For this review, take the finished solid that the model builds, in its own axes (mm). Face numbers are marked on the shaded views. A direction names the side the tool comes from. Coordinates: 2 decimals unless noted, no trailing zeros. Order: outer loops, then holes, each group sorted by start corner. A loop starts at its lowest first (then second) coordinate and runs counter-clockwise, first axis right, second up. Notation, with made-up numbers: (3, 64.5) -> (43, 64.5) arc R19 cw to (43, 98.5) -> close; hole circle Ø8 at (87, 21). An arc over 180 degrees is marked (long way). Answer as a JSON object with one key per item and string values. Group by question number.
1) For pin 1 (3 mm diameter, centred on y = 22.5, z = 13.5, fed in from +X); pin 2 (16.5 mm diameter, centred on y = 17, z = -3, fed in from +X); pin 3 (6 mm diameter, centred on x = -4, z = 11, fed in from -Y); pin 4 (10 mm diameter, centred on x = -21, y = 1, fed in from -Z), all flat-tipped, find the tip position at first contact; note any pin that passes through.
2) Draft analysis for pull direction X (two halves, no side actions). For the marked faces 1, 2, 3 and 4, state which applies: +X half, -X half, draft (parallel to the pull), parting line (faces both ways), or undercut.
3) Add section C-C, the plane x = 27. Write out the cut boundary in (y, z), then the cut area to 3 significant figures.
4) Add section D-D, the plane x = 12. Write out the cut boundary in (y, z), then the cut area to 3 significant figures.
5) Add section B-B, the plane y = 15. Write out the cut boundary in (x, z), then the cut area to 3 significant figures.
6) Wall thickness on L1, parallel to X at y = -7, z = 1; L2, parallel to Y at x = 28.25, z = 0; L3, parallel to Y at x = -1, z = 0: over which ranges is each line inside the solid? List them lowest first.
7) Machinability: for the marked faces 5, 6 and 7, which of the approach directions +Z, -Z, +X, -X, +Y, -Y give a long, thin tool a straight path to every point of the face, cutting with its end or side? Answer none if there is none.
8) Add section A-A, the plane z = 0. Write out the cut boundary in (x, y), then the cut area to 3 significant figures.
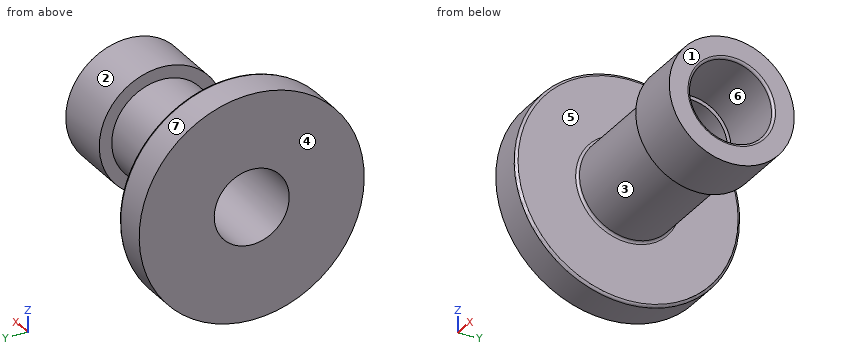
from build123d import *

# Parameters (mm, degrees)
HOLE1_D     = 30
HOLE2_D     = 33
HOLE2_DEPTH = 30
FILLET1_R   = 1


with BuildPart() as part:
    # Sketch1 → Revolve1 (revolve)
    with BuildSketch(Plane.XY, mode=Mode.PRIVATE) as revolve1_sk:
        Polygon((-44.2, 15), (-44.2, 60), (-30, 60), (-30, 35), (20.2, 35), (20.2, 40), (44.2, 40), (44.2, 15), align=None)
    revolve(revolve1_sk.sketch.rotate(Axis((44.2, 15, 0), (-1, 0, 0)), 90), axis=Axis((44.2, 15, 0), (-1, 0, 0)))

    # Hole1 (through all)
    with Locations(Plane(origin=(44.2, 0, 0), x_dir=(0, 0, -1), z_dir=(1, 0, 0))):
        with Locations((0, 15)):
            Hole(HOLE1_D / 2)

    # Hole2
    with Locations(Plane(origin=(44.2, 0, 0), x_dir=(0, 0, -1), z_dir=(1, 0, 0))):
        with Locations((0, 15)):
            Hole(HOLE2_D / 2, depth=HOLE2_DEPTH)

    # Fillet1
    fillet1_edges = [part.edges().sort_by_distance(p)[0] for p in [
        (44.2, 15, -16.5),
        (-30, 15, 20),
        (-30, 15, 45),
    ]]
    fillet(fillet1_edges, radius=FILLET1_R)


solid = part.part
Output values:
{
 "1": {"pin 1": "stops at x = 44.03", "pin 2": "passes through", "pin 3": "stops at y = -3.33", "pin 4": "stops at z = -17.86"},
 "2": {"face 1": "+X half", "face 2": "draft", "face 3": "undercut", "face 4": "-X half"},
 "3": {"outline": "circle Ø50 at (15, 0); hole circle Ø33 at (15, 0)", "area": "1,110 mm²"},
 "4": {"outline": "circle Ø40 at (15, 0); hole circle Ø30 at (15, 0)", "area": "550 mm²"},
 "5": {"outline": "(-44.2, -45) -> (-31, -45) arc R1 ccw to (-30, -44) -> (-30, -21) arc R1 cw to (-29, -20) -> (20.2, -20) -> (20.2, -25) -> (44.2, -25) -> (44.2, -17.5) arc R1 ccw to (43.2, -16.5) -> (14.2, -16.5) -> (14.2, -15) -> (-44.2, -15) -> close; (-44.2, 15) -> (14.2, 15) -> (14.2, 16.5) -> (43.2, 16.5) arc R1 ccw to (44.2, 17.5) -> (44.2, 25) -> (20.2, 25) -> (20.2, 20) -> (-29, 20) arc R1 cw to (-30, 21) -> (-30, 44) arc R1 ccw to (-31, 45) -> (-44.2, 45) -> close", "area": "1,740 mm²"},
 "6": {"L1": "x = -44.2 to -30, 20.2 to 44.2", "L2": "y = -10 to -1.5, 31.5 to 40", "L3": "y = -5 to 0, 30 to 35"},
 "7": {"face 5": "none", "face 6": "+X", "face 7": "+X, -X"},
 "8": {"outline": "(-44.2, -30) -> (-31, -30) arc R1 ccw to (-30, -29) -> (-30, -6) arc R1 cw to (-29, -5) -> (20.2, -5) -> (20.2, -10) -> (44.2, -10) -> (44.2, -2.5) arc R1 ccw to (43.2, -1.5) -> (14.2, -1.5) -> (14.2, 0) -> (-44.2, 0) -> close; (-44.2, 30) -> (14.2, 30) -> (14.2, 31.5) -> (43.2, 31.5) arc R1 ccw to (44.2, 32.5) -> (44.2, 40) -> (20.2, 40) -> (20.2, 35) -> (-29, 35) arc R1 cw to (-30, 36) -> (-30, 59) arc R1 ccw to (-31, 60) -> (-44.2, 60) -> close", "area": "1,740 mm²"}
}
